Autodesk Inventor part; units mm, degrees
ref_plane "YZ Plane" through (0, 0, 0) normal (1, 0, 0) x (0, 1, 0)
ref_plane "XZ Plane" through (0, 0, 0) normal (0, 1, 0) x (-1, 0, 0)
ref_plane "XY Plane" through (0, 0, 0) normal (0, 0, 1) x (1, 0, 0)
sketch "Sketch1" plane through (0, 0, 0) normal (1, 0, 0) x (0, 1, 0)
  circle A0 centre (99.0555, 7.2619) radius 1.6
  line L0 (99.0555, 7.2619) -> (-50.9445, 7.2619) construction
  line L1 (99.0555, 7.2619) -> (249.0555, 7.2619) construction
  circle A1 centre (-50.9445, 7.2619) radius 1.6
  circle A2 centre (99.0555, 7.2619) radius 1.6
  line L2 (99.0305, 11.4695) -> (119.0305, 11.4695)
  line L3 (119.0305, 11.4695) -> (119.0305, -11.2305)
  line L4 (119.0305, 11.4695) -> (141.7305, 11.4695) construction
  line L5 (119.0305, -11.2305) -> (-70.9695, -11.2305)
  line L6 (-70.9695, -11.2305) -> (-70.9695, 11.4695)
  line L7 (-70.9695, 11.4695) -> (99.0305, 11.4695)
  point P0 (0, 0)
  dimension "d0" = 150
  dimension "d1" = 180
  dimension "d2" = 3.2
  dimension "d3" = 3.2
  dimension "d4" = 20
  dimension "d5" = 22.7
  dimension "d6" = 90
  dimension "d7" = 190
  dimension "d8" = 90
  dimension "d9" = 22.7
  dimension "d10" = 90
extrude "Extrusion1" add sketch "Sketch1" along normal blind 2.6
properties part number "Template-Fixture-Side"
Here's how the part is built. I have some questions about the finished solid (model axes, mm). Coordinates: 2 decimals unless noted, no trailing zeros. Answer as a JSON object with one key per item and string values. Group by question number.
(1) If we mould it in two halves opening along Y, with no side actions, what happens to faces 1 (the face through (1.28, 100.58, 6.78)), 2 (the face through (2.6, 23, 0)), 3 (the face through (1.28, -49.42, 6.78))? For each: released by +Y, released by -Y, zero draft, split by the parting line, or undercut.
(2) I need wall thicknesses on probe 1 along Y at (x, z) = (1.05, 8). Which ranges of the line are inside material? Lowest first, please.
(3) For pin 1 (1.9 mm diameter, centred on y = 99.06, z = 7.26, fed in from -X), with a flat end and sliding along its axis, tell me the tip position at first contact or that it passes through.
Values found:
{
 "1": {"face 1": "undercut", "face 2": "zero draft", "face 3": "undercut"},
 "2": {"probe 1": "y = -70.97 to -52.36, -49.52 to 97.64, 100.48 to 119.03"},
 "3": {"pin 1": "passes through"}
}
